Could you check a few things on this model? Use its own coordinates, in mm. Give positions to 0.01 mm unless a question says otherwise; leave off trailing zeros. Write each loop counter-clockwise with the first axis right and the second up, starting at its lowest first coordinate (ties: lowest second). Pieces come first, ordered by that corner, then holes. Notation, with made-up numbers: (89, -10) - (117, -10) arc R25 cw to (117, 2) - close; hole circle Ø5 at (58.5, 56). An arc over 180 degrees is marked (long way). Write item = value, one per line.
Autodesk Fusion 360 part; units mm, degrees
sketch "Sketch1" plane through (0, 0, 0) normal (1, 0, 0) x (0, 1, 0) in component "probe_retainer_bracket"
  line L0 (9.35, 4.1) -> (-9.35, 4.1)
  line L1 (-9.35, 4.1) -> (-9.35, -4.1)
  line L2 (-9.35, -4.1) -> (9.35, -4.1)
  line L3 (9.35, -4.1) -> (9.35, 4.1)
  line L4 (9.35, 4.1) -> (-9.35, -4.1) construction
  line L5 (-9.35, 4.1) -> (9.35, -4.1) construction
  circle A0 centre (-5.25, -0.0082) radius 2.4
  line L6 (0, 0) -> (-10.0428, -0.0157) construction
  line L7 (0, 0) -> (0, 6) construction
  circle A1 centre (5.25, -0.0082) radius 2.4
  dimension "d1" = 18.7
  dimension "d2" = 8.2
  dimension "d3" = 4.8
  dimension "d4" = 10.5
extrude "Extrude1" add sketch "Sketch1" along normal mid plane 4 in component "probe_retainer_bracket"
fillet "Fillet1" radius 2 4 edges at (0, -9.35, 4.1) (0, 9.35, 4.1) (0, -9.35, -4.1) (0, 9.35, -4.1) in component "probe_retainer_bracket"
fillet "Fillet2" radius 1 8 edges at (2, -8.7642, 3.5142) (2, -9.35, 0) (2, -8.7642, -3.5142) (2, 0, -4.1) (2, 8.7642, -3.5142) (2, 9.35, 0) (2, 8.7642, 3.5142) (2, 0, 4.1) in component "probe_retainer_bracket"
component "probe_retainer_bracket" placed x (1, 0, 0) y (0, 1, 0) z (0, 0, 1) at (0, 0, 0)
1. For pin 1 (1.5 mm diameter, centred on x = 1.5, y = 5, fed in from -Z), with a flat end and sliding along its axis, tell me the tip position at first contact or that it passes through.
Filled sheet:
pin_1 = -4.1
2. I need wall thicknesses on line 1 (Y direction, x = 1.5, z = -0.5); line 2 (Z direction, x = 1.1, y = -5.25); line 3 (Y direction, x = 1.65, z = -0.25). Which ranges of each line are inside material? Lowest first, please.
Filled sheet:
line_1 = -9.22 to -7.6, -2.9 to 2.9, 7.6 to 9.22
line_2 = -4.09 to -2.41, 2.39 to 4.09
line_3 = -9.11 to -7.64, -2.86 to 2.86, 7.64 to 9.11
3. If we section it at A-A, the plane y = -5.25: Please give me the cut outline in (x, z), and give its area (3 significant figures).
Filled sheet:
outline = (-2, -4.1) - (1, -4.1) arc R1 ccw to (2, -3.1) - (2, -2.41) - (-2, -2.41) - close; (-2, 2.39) - (2, 2.39) - (2, 3.1) arc R1 ccw to (1, 4.1) - (-2, 4.1) - close
area = 13.2 mm2
4. Thinking about a two-plate mould opening in Y: for faces 1 (the face through (-0.028, -5.77, 2.335)), 2 (the face through (-0.52, 8.78, -3.5)), 3 (the face through (-1, 0, -4.1)), which applies, pulls with the +Y half, pulls with the -Y half, needs draft (parallel to the pull), parting line crosses it, or undercut?
Filled sheet:
face_1 = undercut
face_2 = pulls with the +Y half
face_3 = needs draft
5. If we section it at C-C, the plane x = -0.9: Please give me the cut outline in (y, z).
Filled sheet:
outline = (-9.35, -2.1) arc R2 ccw to (-7.35, -4.1) - (7.35, -4.1) arc R2 ccw to (9.35, -2.1) - (9.35, 2.1) arc R2 ccw to (7.35, 4.1) - (-7.35, 4.1) arc R2 ccw to (-9.35, 2.1) - close; hole circle Ø4.8 at (-5.25, -0.01); hole circle Ø4.8 at (5.25, -0.01)
6. If we section it at D-D, the plane y = 5: Please give me the cut outline in (x, z).
Filled sheet:
outline = (-2, -4.1) - (1, -4.1) arc R1 ccw to (2, -3.1) - (2, -2.4) - (-2, -2.4) - close; (-2, 2.38) - (2, 2.38) - (2, 3.1) arc R1 ccw to (1, 4.1) - (-2, 4.1) - close
7. If we section it at B-B, the plane z = 0.75: Please give me the cut outline in (x, y), and give its area (3 significant figures).
Filled sheet:
outline = (-2, -9.35) - (1, -9.35) arc R1 ccw to (2, -8.35) - (2, -7.53) - (-2, -7.53) - close; (-2, -2.97) - (2, -2.97) - (2, 2.97) - (-2, 2.97) - close; (-2, 7.53) - (2, 7.53) - (2, 8.35) arc R1 ccw to (1, 9.35) - (-2, 9.35) - close
area = 37.9 mm2
